Part model, mm, in its own coordinate system. Face numbers are marked on the shaded views. A direction names the side the tool comes from. Coordinates: 2 decimals unless noted, no trailing zeros. Order: outer loops, then holes, each group sorted by start corner. A loop starts at its lowest first (then second) coordinate and runs counter-clockwise, first axis right, second up.
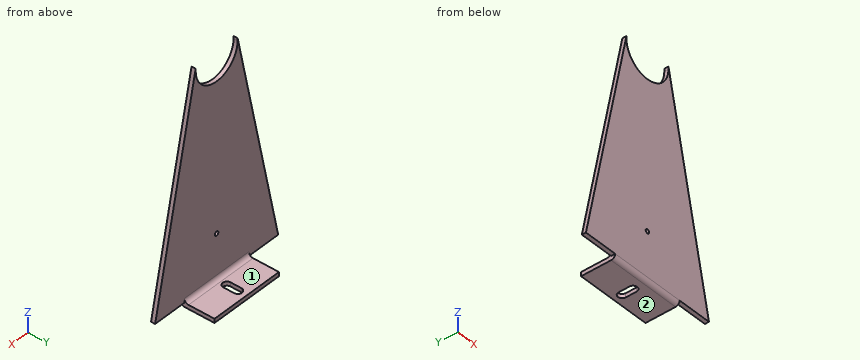
from build123d import *

# Parameters (mm, degrees)
F0_R     = 1.5
F1_DEPTH = 3
F2_W     = 55
F2_H     = 3
F3_DEPTH = 25
F4_R     = 3
F6_DEPTH = 163.1321276775


with BuildPart() as f1:
    # F0 (on Front) → F1 (new body)
    with BuildSketch(Plane.XZ):
        with BuildLine():
            Line((454.8277321524, 574.7700988736), (454.8277321524, 576.6820907487))
            Line((454.8277321524, 576.6820907487), (420.231500864, 416.5509630712))
            Line((420.231500864, 416.5509630712), (495.9500458773, 416.5509630712))
            Line((495.9500458773, 416.5509630712), (525.231500864, 416.5509630712))
            Line((525.231500864, 416.5509630712), (490.6352695757, 576.6820907487))
            Line((490.6352695757, 576.6820907487), (490.6352695757, 574.7700988736))
            ThreePointArc((490.6352695757, 574.7700988736), (472.731500864, 556.866330162), (454.8277321524, 574.7700988736))
        make_face()
        with Locations((472.731500864, 449.0509630712)):
            Circle(F0_R, mode=Mode.SUBTRACT)
    extrude(amount=F1_DEPTH)

    # F2 (on face) → F3 (join)
    with BuildSketch(Plane.XZ.offset(3)):
        with Locations((472.731500864, 415.0509630712)):
            Rectangle(F2_W, F2_H)
    extrude(amount=-F3_DEPTH)

    # F4
    f4_edges = [f1.edges().sort_by_distance(p)[0] for p in [
        (472.731501, -3, 413.550963),
        (472.731501, 0, 416.550963),
    ]]
    fillet(f4_edges, radius=F4_R)

    # F5 (on face) → F6 (cut, through all)
    with BuildSketch(Plane(origin=(0, 0, 413.5509630712), x_dir=(1, 0, 0), z_dir=(0, 0, -1))):
        with BuildLine():
            Line((475.731500864, -15.5), (475.731500864, -7.5))
            ThreePointArc((475.731500864, -7.5), (472.731500864, -4.5), (469.731500864, -7.5))
            Line((469.731500864, -7.5), (469.731500864, -15.5))
            ThreePointArc((469.731500864, -15.5), (472.731500864, -18.5), (475.731500864, -15.5))
        make_face()
    extrude(amount=-F6_DEPTH, mode=Mode.SUBTRACT)


solid = f1.part
Q1. Which spindle directions (+Z, -Z, +X, -X, +Y, -Y) get a long thin tool onto all of the face, cutting with end or side? Do the marked faces 1 and 2. Say none if no direction does.
Results list:
face 1: +Z, +X, -X, +Y
face 2: -Z, +X, -X, +Y, -Y
Q2. Cut at B-B on z = 564. Write the cut outline in (x, y), and give its area (3 significant figures).
Results list:
outline: (452.09, -3) - (458.43, -3) - (458.43, 0) - (452.09, 0) - close; (487.03, -3) - (493.38, -3) - (493.38, 0) - (487.03, 0) - close
area: 38.0 mm2
Q3. Wall check: line 1 along Y through (x, z) = (478, 455.5); line 2 along Z through (x, y) = (457, 17.5); line 3 along Z through (x, y) = (484, -1). Give the ranges that are in metal, low to high.
Results list:
line 1: y = -3 to 0
line 2: z = 413.55 to 416.55
line 3: z = 413.72 to 560.86
Q4. Cut at A-A on y = 11.75. Write the cut outline in (x, z), and give its area (3 significant figures).
Results list:
outline: (445.23, 413.55) - (469.73, 413.55) - (469.73, 416.55) - (445.23, 416.55) - close; (475.73, 413.55) - (500.23, 413.55) - (500.23, 416.55) - (475.73, 416.55) - close
area: 147 mm2
Q5. Cut at D-D on z = 536. Write the cut outline in (x, y).
Results list:
outline: (446.04, -3) - (499.42, -3) - (499.42, 0) - (446.04, 0) - close
Q6. Pin check, flat tips, straight feed: pin 1 Ø2 at (y, z) = (-2, 575.5) entering from +X; pin 2 Ø3 at (y, z) = (7, 417) entering from -X; pin 3 Ø15 at (x, y) = (483.5, 8.5) entering from +Z; pin 4 Ø5 at (x, y) = (473, 9) entering from -Z. Stop position of each tip, or through.
Results list:
pin 1: stops at x = 491.11
pin 2: stops at x = 445.23
pin 3: stops at z = 417.31
pin 4: passes through
Q7. Cut at C-C on x = 478. Write the cut outline in (y, z), and give its area (3 significant figures).
Results list:
outline: (-3, 416.55) arc R3 ccw to (0, 413.55) - (22, 413.55) - (22, 416.55) - (3, 416.55) arc R3 cw to (0, 419.55) - (0, 557.66) - (-3, 557.66) - close
area: 498 mm2
